Input: part model. Units: mm. Frame: model coordinates. A direction names the side the tool comes from. Give positions to 0.01 mm unless a question says otherwise; leave off trailing zeros. Write each loop counter-clockwise with the first axis right and the second up, starting at its lowest first coordinate (ties: lowest second). Pieces come first, ordered by that corner, then holes. Notation, with made-up numbers: M 12,42 L 34,42 A33 cw 34,73 Z; hole C -16.5,33 d6. An arc over 180 degrees is marked long. Use CSV: the item, a comma, the result in double quotes. Start each with the question number.
from build123d import *

# Parameters (mm, degrees)
SKETCH1_W           = 40
SKETCH1_H           = 30
BOSS_EXTRUDE1_DEPTH = 33.2
SKETCH2_R           = 4.205
CUT_EXTRUDE1_DEPTH  = 55.103973976
CUT_EXTRUDE2_DEPTH  = 3.12
SKETCH4_W           = 60
SKETCH4_H           = 5
BOSS_EXTRUDE2_DEPTH = 40
FILLET1_R           = 5
SKETCH5_W           = 20
SKETCH5_H           = 1.05
CUT_EXTRUDE3_DEPTH  = 10


with BuildPart() as part:
    # Sketch1 → Boss-Extrude1 (new body)
    with BuildSketch(Plane(origin=(0, 0, 0), x_dir=(1, 0, 0), z_dir=(0, 1, 0))):
        Rectangle(SKETCH1_W, SKETCH1_H)
    extrude(amount=BOSS_EXTRUDE1_DEPTH)

    # Sketch2 → Cut-Extrude1 (cut, through all)
    with BuildSketch(Plane.ZY.offset(20)):
        with Locations((0, 33.2)):
            Circle(SKETCH2_R)
    extrude(amount=-CUT_EXTRUDE1_DEPTH, mode=Mode.SUBTRACT)

    # Sketch3 → Cut-Extrude2 (cut)
    with BuildSketch(Plane(origin=(0, 33.2, 0), x_dir=(1, 0, 0), z_dir=(0, 1, 0))):
        Polygon((2.020725942, 6.5), (4.041451884, 10), (2.020725942, 13.5), (-2.020725942, 13.5), (-4.041451884, 10), (-2.020725942, 6.5), align=None)
    cut_extrude2 = extrude(amount=-CUT_EXTRUDE2_DEPTH, mode=Mode.SUBTRACT)

    # Mirror1: Cut-Extrude2 across plane
    add(cut_extrude2.mirror(Plane.XY), mode=Mode.SUBTRACT)

    # Sketch4 → Boss-Extrude2 (add)
    with BuildSketch(Plane(origin=(20, 0, 0), x_dir=(0, 0, -1), z_dir=(1, 0, 0))):
        with Locations((0, 2.5)):
            Rectangle(SKETCH4_W, SKETCH4_H)
    extrude(amount=-BOSS_EXTRUDE2_DEPTH)

    # Fillet1
    fillet1_edges = [part.edges().sort_by_distance(p)[0] for p in [
        (0, 5, -15),
        (0, 5, 15),
    ]]
    fillet(fillet1_edges, radius=FILLET1_R)

    # Sketch5 → Cut-Extrude3 (cut)
    with BuildSketch(Plane.ZY.offset(20)):
        with Locations((0, 33.2)):
            Rectangle(SKETCH5_W, SKETCH5_H)
    extrude(amount=-CUT_EXTRUDE3_DEPTH, mode=Mode.SUBTRACT)


solid = part.part
Q1. First-contact query: pin 1 Ø7 at (x, y) = (7.5, 24.5) entering from -Z; pin 2 Ø18.5 at (x, y) = (1.5, 22.5) entering from +Z; pin 3 Ø5 at (x, y) = (6.5, 8.5) entering from +Z. Flat tips, straight axial feed; report the tip coordinate or a pass-through.
Q2. Section B-B, the plane z = -25.5. Return the cut outline in (x, y).
Q3. Set-up query: faces 1 (the flat face through (0, 5, 25)), 2 (the flat face through (0, 2, 30)), 3 (the flat face through (3.045, 31.662, 11.726)), 4 (the flat face through (0, 2, -30)), 5 (the flat face through (-15, 32.675, 7)). Return all of +Z, -Z, +X, -X, +Y, -Y with unobstructed straight access to the full face (end or side cutting, diameter ignored); none if empty.
Q4. Pull-direction query (X, two-part tool) for faces 6 (the flat face through (-20, 17, 0)), 7 (the flat face through (0, 32, -6.5)), 8 (the cylindrical face through (-0.28, 28.996, -0.092)); classes: released by +X, released by -X, zero draft, split by the parting line, or undercut.
Q5. Material intervals for L1, parallel to Z at x = -13, y = 24; L2, parallel to Y at x = -14.5, z = 18; L3, parallel to Z at x = -16, y = 6, sorted ascending. Write a range as [from, to].
Q6. Section D-D, the plane z = 0. Return the cut outline in (x, y) (3 decimals), and give its area (3 significant figures).
Q7. Section A-A, the plane x = -18. Return the cut outline in (y, z) (3 decimals), and give its area (3 significant figures).
Q8. Section C-C, the plane x = 17.5. Return the cut outline in (y, z) (3 decimals), and give its area (3 significant figures).
Check result:
1,pin 1,"stops at z = -15"
1,pin 2,"stops at z = 15"
1,pin 3,"stops at z = 17"
2,outline,"M -20,0 L 20,0 L 20,5 L -20,5 Z"
3,face 1,"+Z, +X, -X, +Y"
3,face 2,"+Z, +X, -X, +Y, -Y"
3,face 3,"+Y"
3,face 4,"-Z, +X, -X, +Y, -Y"
3,face 5,"-X, +Y"
4,face 6,"released by -X"
4,face 7,"undercut"
4,face 8,"zero draft"
5,L1,"z = [-15, 15]"
5,L2,"y = [0, 5.42]"
5,L3,"z = [-17, 17]"
6,outline,"M -20,0 L 20,0 L 20,28.995 L -20,28.995 Z"
6,area,"1,160 mm²"
7,outline,"M 0,-30 L 5,-30 L 5,-20 A5 cw 10,-15 L 33.2,-15 L 33.2,-10 L 32.675,-10 L 32.675,-4.172 A4.205 cw 32.675,4.172 L 32.675,10 L 33.2,10 L 33.2,15 L 10,15 A5 cw 5,20 L 5,30 L 0,30 Z"
7,area,"1,120 mm²"
8,outline,"M 0,-30 L 5,-30 L 5,-20 A5 cw 10,-15 L 33.2,-15 L 33.2,-4.205 A4.205 cw 33.2,4.205 L 33.2,15 L 10,15 A5 cw 5,20 L 5,30 L 0,30 Z"
8,area,"1,130 mm²"
